Verification items for this drawing (mm, ordinates from the low corner). Round coordinates to 2 decimals unless told otherwise and drop trailing zeros. Order: outer loops, then holes, each group sorted by start corner. A loop starts at its lowest first (then second) coordinate and runs counter-clockwise, first axis right, second up. Notation, with made-up numbers: M 50,-28 L 79,-28 A16 cw 79,-16 Z; hole C 87,51.5 d8. An arc over 180 degrees is marked long. Return JSON: item names as keys, results as strings. Group by question number.
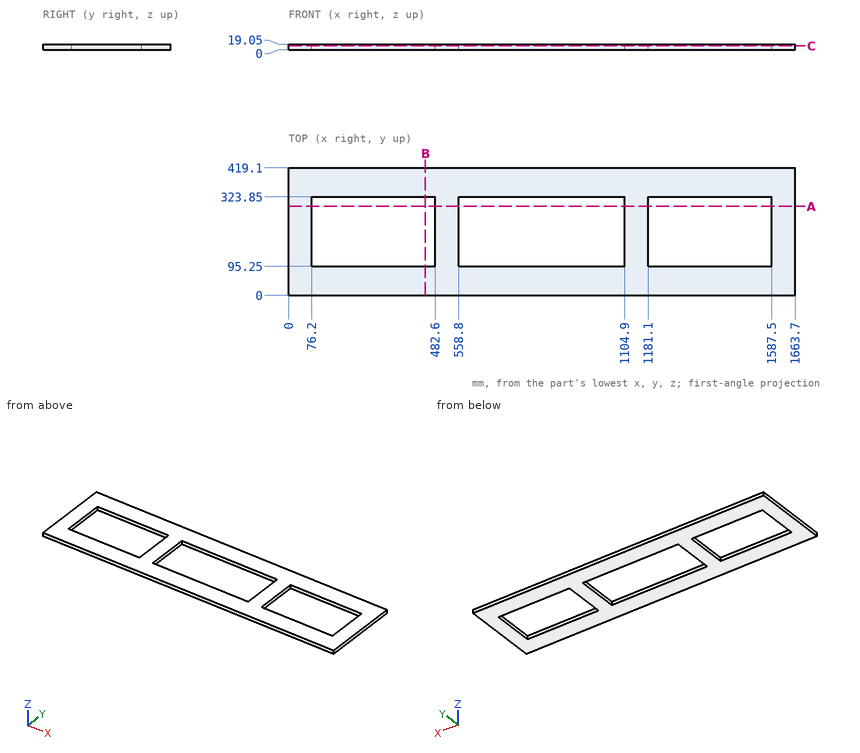
1. Cross-section at B-B (x = 449). Enter the section's corners in (y, z).
2. Cross-section at A-A (y = 292). Enter the section's corners in (x, z), plus the area to 3 significant figures.
3. Cross-section at C-C (z = 13.25). Enter the section's corners in (x, y), plus the area to 3 significant figures.
4. Thickness scan on line 1 along X through (y, z) = (322, 8.5); line 2 along Y through (x, z) = (948.5, 6.25). Record the ranges inside material, lowest first. Write a range as from..to.
Computed:
{
 "1": {"outline": "M 0,0 L 95.25,0 L 95.25,19.05 L 0,19.05 Z; M 323.85,0 L 419.1,0 L 419.1,19.05 L 323.85,19.05 Z"},
 "2": {"outline": "M 0,0 L 76.2,0 L 76.2,19.05 L 0,19.05 Z; M 482.6,0 L 558.8,0 L 558.8,19.05 L 482.6,19.05 Z; M 1104.9,0 L 1181.1,0 L 1181.1,19.05 L 1104.9,19.05 Z; M 1587.5,0 L 1663.7,0 L 1663.7,19.05 L 1587.5,19.05 Z", "area": "5,810 mm²"},
 "3": {"outline": "M 0,0 L 1663.7,0 L 1663.7,419.1 L 0,419.1 Z; hole M 76.2,95.25 L 482.6,95.25 L 482.6,323.85 L 76.2,323.85 Z; hole M 558.8,95.25 L 1104.9,95.25 L 1104.9,323.85 L 558.8,323.85 Z; hole M 1181.1,95.25 L 1587.5,95.25 L 1587.5,323.85 L 1181.1,323.85 Z", "area": "387,000 mm²"},
 "4": {"line 1": "x = 0..76.2, 482.6..558.8, 1104.9..1181.1, 1587.5..1663.7", "line 2": "y = 0..95.25, 323.85..419.1"}
}
